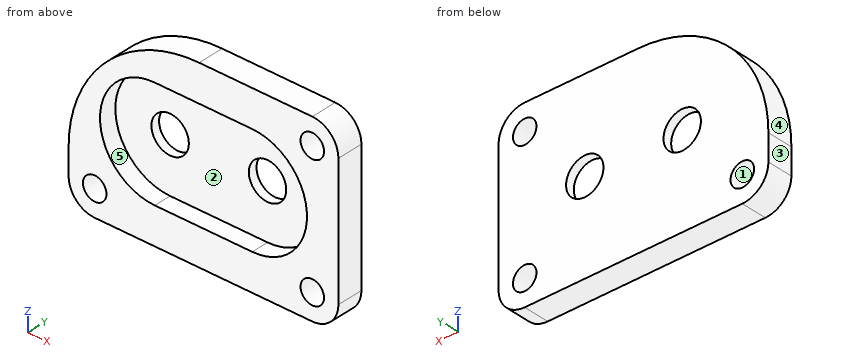
from build123d import *

# Parameters (mm, degrees)
SKETCH1_R           = 2.15
SKETCH1_R_2         = 1.35
BOSS_EXTRUDE1_DEPTH = 3
CUT_EXTRUDE1_DEPTH  = 2


with BuildPart() as part:
    # Sketch1 → Boss-Extrude1 (new body)
    with BuildSketch(Plane(origin=(0, 0, 0), x_dir=(1, 0, 0), z_dir=(0, 1, 0))):
        with BuildLine():
            Line((5.095, -10.5), (18.095, -10.5))
            ThreePointArc((18.095, -10.5), (20.216320344, -9.621320344), (21.095, -7.5))
            Line((21.095, -7.5), (21.095, 7.5))
            ThreePointArc((21.095, 7.5), (20.216320344, 9.621320344), (18.095, 10.5))
            Line((18.095, 10.5), (-6.905, 10.5))
            ThreePointArc((-6.905, 10.5), (-9.026320344, 9.621320344), (-9.905, 7.5))
            Line((-9.905, 7.5), (-9.905, 4.5))
            ThreePointArc((-9.905, 4.5), (-5.511601718, -6.106601718), (5.095, -10.5))
        make_face()
        Circle(SKETCH1_R, mode=Mode.SUBTRACT)
        with Locations((11.19, 0)):
            Circle(SKETCH1_R, mode=Mode.SUBTRACT)
        with Locations((-6.905, 7.5)):
            Circle(SKETCH1_R_2, mode=Mode.SUBTRACT)
        with Locations((18.095, 7.5)):
            Circle(SKETCH1_R_2, mode=Mode.SUBTRACT)
        with Locations((18.095, -7.5)):
            Circle(SKETCH1_R_2, mode=Mode.SUBTRACT)
    extrude(amount=BOSS_EXTRUDE1_DEPTH)

    # Sketch2 → Cut-Extrude1 (cut)
    with BuildSketch(Plane.XZ):
        with BuildLine():
            Line((0, 6.29609527), (11.19, 6.29609527))
            ThreePointArc((11.19, 6.29609527), (17.48609527, 0), (11.19, -6.29609527))
            Line((11.19, -6.29609527), (0, -6.29609527))
            ThreePointArc((0, -6.29609527), (-6.29609527, 0), (0, 6.29609527))
        make_face()
    extrude(amount=-CUT_EXTRUDE1_DEPTH, mode=Mode.SUBTRACT)


solid = part.part
Verification items for the finished model (mm, model axes). Face numbers are marked on the shaded views. A direction names the side the tool comes from. Give positions to 0.01 mm unless a question says otherwise; leave off trailing zeros. Order: outer loops, then holes, each group sorted by start corner. A loop starts at its lowest first (then second) coordinate and runs counter-clockwise, first axis right, second up. Notation, with made-up numbers: M -34,29 L -11,29 A21 cw -11,46 Z; hole C 15.25,85 d11. An arc over 180 degrees is marked long. Answer as a JSON object with one key per item and string values. Group by question number.
1) Cross-section at B-B (z = 0). Enter the section's corners in (x, y) (3 decimals), then the cut area to 3 significant figures.
2) Cross-section at A-A (y = 1.1). Enter the section's corners in (x, z) (3 decimals), then the cut area to 3 significant figures.
3) Cross-section at D-D (z = -2.75). Enter the section's corners in (x, y) (3 decimals), then the cut area to 3 significant figures.
4) Access from +Z, -Z, +X, -X, +Y, -Y to the whole of each face (thin tool, end or side, straight path). Record for the marked faces 1 and 2.
5) Scan lines: line 1 along X through (y, z) = (0.7, -7.5) (3 decimals); line 2 along Z through (x, y) = (11.19, 2.5); line 3 along Z through (x, y) = (8.5, 0.25). Record each from-to range of solid material in increasing order. Write a range as [from, to].
6) Mould release check, pull along Z, two halves, no side actions. Record for the marked faces 3, 4 and 5: released by +Z, released by -Z, zero draft, split by the parting line, or undercut.
7) Depth check by flat-ended pin: pin 1 Ø7 at (x, z) = (11.19, 0) entering from -Y. Enter the tip coordinate at first touch or a pass-through.
8) Cross-section at C-C (x = -5). Enter the section's corners in (y, z), then the cut area to 3 significant figures.
Result sheet:
{
 "1": {"outline": "M -9.214,0 L -6.296,0 L -6.296,2 L -2.15,2 L -2.15,3 L -9.214,3 Z; M 2.15,2 L 9.04,2 L 9.04,3 L 2.15,3 Z; M 13.34,2 L 17.486,2 L 17.486,0 L 21.095,0 L 21.095,3 L 13.34,3 Z", "area": "34.8 mm2"},
 "2": {"outline": "M -9.905,-7.5 A3 ccw -6.905,-10.5 L 18.095,-10.5 A3 ccw 21.095,-7.5 L 21.095,7.5 A3 ccw 18.095,10.5 L 5.095,10.5 A15 ccw -9.905,-4.5 Z; hole C -6.905,-7.5 d2.7; hole M 0,-6.296 L 11.19,-6.296 A6.296 ccw 11.19,6.296 L 0,6.296 A6.296 ccw Z; hole C 18.095,-7.5 d2.7; hole C 18.095,7.5 d2.7", "area": "314 mm2"},
 "3": {"outline": "M -9.803,0 L -5.664,0 L -5.664,2 L 16.854,2 L 16.854,0 L 21.095,0 L 21.095,3 L -9.803,3 Z", "area": "47.7 mm2"},
 "4": {"face 1": "+Y, -Y", "face 2": "-Y"},
 "5": {"line 1": "x = [-9.905, -8.255], [-5.555, 16.745], [19.445, 21.095]", "line 2": "z = [-10.5, -2.15], [2.15, 10.5]", "line 3": "z = [-10.5, -6.3], [6.3, 10.5]"},
 "6": {"face 3": "zero draft", "face 4": "released by +Z", "face 5": "undercut"},
 "7": {"pin 1": "stops at y = 2"},
 "8": {"outline": "M 0,-10.5 L 3,-10.5 L 3,6.59 L 0,6.59 L 0,3.83 L 2,3.83 L 2,-3.83 L 0,-3.83 Z", "area": "36.0 mm2"}
}
